Check sheet for the modelled part. Datum: model origin and axes. Units: mm. A direction names the side the tool comes from. Round coordinates to 2 decimals unless told otherwise and drop trailing zeros. Write each loop counter-clockwise with the first axis right and the second up, starting at its lowest first coordinate (ties: lowest second). Pieces come first, ordered by that corner, then holes. Notation, with made-up numbers: (-25.75, 4.25) - (-18.75, 4.25) arc R19 cw to (-18.75, 18.25) - close; hole circle Ø8 at (-29, -7). An arc over 180 degrees is marked (long way). Use one line per item in the form item = value. Start each with the question number.
1) Gauge pin test, flat ends, axial feed: P1, Ø3, axis at x = -61, y = 31, coming from the +Z side; P2, Ø2, axis at x = 37, z = 55, coming from the +Y side; P3, Ø1.5, axis at y = 27.5, z = 45, coming from the +X side. Record the tip position at first contact, or that the pin passes through.
2) Draft check along X on faces 6 (the face through (-9, 51, 0)), 7 (the face through (-0.975, -74.994, 9.86)), 8 (the face through (92.136, 25.524, 9.86)). Enter one of: +X half, -X half, draft (parallel to the pull), parting line (faces both ways), or undercut.
3) Scan lines: probe 1 along Y at (x, z) = (-150, 24); probe 2 along X at (y, z) = (26.5, 23); probe 3 along Z at (x, y) = (129, 21.5). Record each from-to range of solid material in increasing order.
4) Section check C-C (z = 46). Record the boundary of the cut face in (x, y), then the cut area to 3 significant figures.
5) Section check B-B (x = 0). Record the boundary of the cut face in (y, z).
6) Section check D-D (x = 150). Record the boundary of the cut face in (y, z).
7) Section check A-A (y = 0). Record the boundary of the cut face in (x, z).
8) Set-up check for faces 1 (the face through (-174.5, 5.7, 40)), 2 (the face through (-174.976, 1.099, 19.72)), 3 (the face through (-187.302, -14.442, 19.72)), 4 (the face through (-23, 45, 70)), 5 (the face through (146, 25, 40)): record each of +Z, -Z, +X, -X, +Y, -Y from which the full face is reachable in a straight line by a thin tool's end or side.
from build123d import *

# Parameters (mm, degrees)
SKETCH1_R           = 75
SKETCH1_R_2         = 60
BOSS_EXTRUDE4_DEPTH = 20
SKETCH1_5_R         = 40
SKETCH1_5_R_2       = 25
BOSS_EXTRUDE5_DEPTH = 40
SKETCH1_6_R         = 40
SKETCH1_6_R_2       = 25
BOSS_EXTRUDE6_DEPTH = 40
SKETCH1_7_R         = 60
SKETCH1_7_R_2       = 50
BOSS_EXTRUDE7_DEPTH = 70


with BuildPart() as part:
    # Sketch1 → Boss-Extrude4 (new body)
    # profile 1 of 3: a face of its own
    with BuildSketch(Plane.XY):
        with BuildLine():
            ThreePointArc((-60.05, -44.933256058), (-75, 0), (-60.05, 44.933256058))
            ThreePointArc((-60.05, 44.933256058), (-91.612158535, 25.611592996), (-127.814814815, 33.283893377))
            ThreePointArc((-127.814814815, 33.283893377), (-114.733816428, 18.875812467), (-110, 0))
            ThreePointArc((-110, 0), (-114.733816428, -18.875812467), (-127.814814815, -33.283893377))
            ThreePointArc((-127.814814815, -33.283893377), (-91.612158535, -25.611592996), (-60.05, -44.933256058))
        make_face()
    # profile 2 of 3: a face of its own
    with BuildSketch(Plane.XY):
        Circle(SKETCH1_R)
        Circle(SKETCH1_R_2, mode=Mode.SUBTRACT)
    # profile 3 of 3: a face of its own
    with BuildSketch(Plane.XY):
        with BuildLine():
            ThreePointArc((60.05, 44.933256058), (71.164422291, 23.677520985), (75, 0))
            ThreePointArc((75, 0), (71.164422291, -23.677520985), (60.05, -44.933256058))
            ThreePointArc((60.05, -44.933256058), (91.612158535, -25.611592996), (127.814814815, -33.283893377))
            ThreePointArc((127.814814815, -33.283893377), (110, 0), (127.814814815, 33.283893377))
            ThreePointArc((127.814814815, 33.283893377), (91.612158535, 25.611592996), (60.05, 44.933256058))
        make_face()
    extrude(amount=BOSS_EXTRUDE4_DEPTH)

    # Sketch1_5 → Boss-Extrude5 (add)
    with BuildSketch(Plane.XY):
        with Locations(Location((-150, 0, 0), (0, 0, 303.68520838))):
            Circle(SKETCH1_5_R)
        with Locations((-150, 0)):
            Circle(SKETCH1_5_R_2, mode=Mode.SUBTRACT)
    extrude(amount=BOSS_EXTRUDE5_DEPTH)

    # Sketch1_6 → Boss-Extrude6 (add)
    with BuildSketch(Plane.XY):
        with Locations(Location((150, 0, 0), (0, 0, 236.31479162))):
            Circle(SKETCH1_6_R)
        with Locations((150, 0)):
            Circle(SKETCH1_6_R_2, mode=Mode.SUBTRACT)
    extrude(amount=BOSS_EXTRUDE6_DEPTH)

    # Sketch1_7 → Boss-Extrude7 (add)
    with BuildSketch(Plane.XY):
        Circle(SKETCH1_7_R)
        Circle(SKETCH1_7_R_2, mode=Mode.SUBTRACT)
    extrude(amount=BOSS_EXTRUDE7_DEPTH)


solid = part.part
Results are:
q1.P1 = 20
q1.P2 = 48
q1.P3 = 53.71
q2.face_6 = draft
q2.face_7 = parting line
q2.face_8 = undercut
q3.probe_1 = -40 to -25, 25 to 40
q3.probe_2 = -179.96 to -120.04, -53.83 to -42.4, 42.4 to 53.83, 120.04 to 179.96
q3.probe_3 = 0 to 40
q4.outline = circle Ø120 at (0, 0); hole circle Ø100 at (0, 0)
q4.area = 3,460 mm²
q5.outline = (-75, 0) - (-50, 0) - (-50, 70) - (-60, 70) - (-60, 20) - (-75, 20) - close; (50, 0) - (75, 0) - (75, 20) - (60, 20) - (60, 70) - (50, 70) - close
q6.outline = (-40, 0) - (-25, 0) - (-25, 40) - (-40, 40) - close; (25, 0) - (40, 0) - (40, 40) - (25, 40) - close
q7.outline = (-190, 0) - (-175, 0) - (-175, 40) - (-190, 40) - close; (-125, 0) - (-50, 0) - (-50, 70) - (-60, 70) - (-60, 20) - (-110, 20) - (-110, 40) - (-125, 40) - close; (50, 0) - (125, 0) - (125, 40) - (110, 40) - (110, 20) - (60, 20) - (60, 70) - (50, 70) - close; (175, 0) - (190, 0) - (190, 40) - (175, 40) - close
q8.face_1 = +Z, -X, +Y, -Y
q8.face_2 = +Z, -Z
q8.face_3 = +Z
q8.face_4 = +Z, +X, -X, +Y, -Y
q8.face_5 = +Z, +X, +Y, -Y
